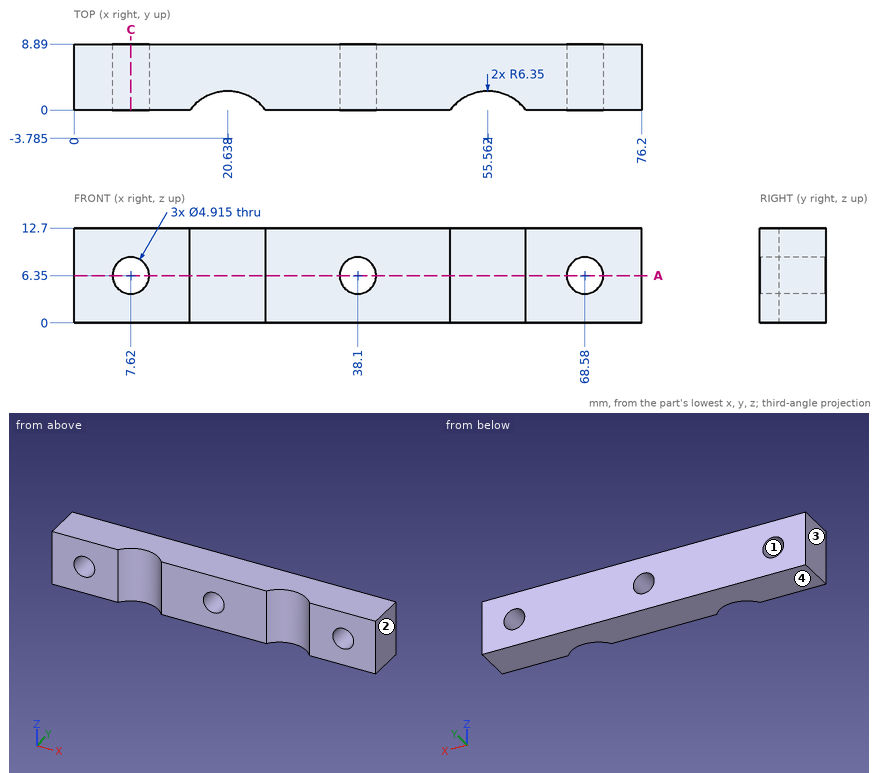
The drawing under review shows one solid part. Ordinate dimensions are in mm from its lowest x, y, z. Give positions to 0.01 mm unless a question says otherwise; leave off trailing zeros. Write each loop counter-clockwise with the first axis right and the second up, starting at its lowest first coordinate (ties: lowest second). Pieces come first, ordered by that corner, then holes.
1. Add section A-A, the plane z = 6.35. Count the separate pieces of the cut face and the enclosed holes in it, plus the area to 3 significant figures.
2. Add section C-C, the plane x = 7.62. Write out the cut boundary in (y, z).
3. Draft analysis for pull direction X (two halves, no side actions). For the marked faces 1, 2, 3 and 4, state which applies: +X half, -X half, draft (parallel to the pull), parting line (faces both ways), or undercut.
4. For P1, Ø5.5, axis at x = 68.58, z = 6.35, coming from the +Y side, flat-tipped, find the tip position at first contact; note if it passes through.
5. Wall thickness on L1, parallel to X at y = 5, z = 6.5; L2, parallel to X at y = 1.5, z = 7.25 (1 decimal); L3, parallel to X at y = 8.75, z = 5 (1 decimal): over which ranges is each line inside the solid? List them lowest first.
Worked answers:
1. separate pieces: 4
1. enclosed holes: 0
1. area: 510 mm2
2. outline: (0, 0) - (8.89, 0) - (8.89, 3.89) - (0, 3.89) - close; (0, 8.81) - (8.89, 8.81) - (8.89, 12.7) - (0, 12.7) - close
3. face 1: undercut
3. face 2: +X half
3. face 3: -X half
3. face 4: draft
4. P1: stops at y = 8.89
5. L1: x = 0 to 5.17, 10.07 to 35.65, 40.55 to 66.13, 71.03 to 76.2
5. L2: x = 0 to 5.3, 9.9 to 17.1, 24.2 to 35.8, 40.4 to 52, 59.1 to 66.3, 70.9 to 76.2
5. L3: x = 0 to 5.6, 9.7 to 36, 40.2 to 66.5, 70.6 to 76.2
